Geometry: final body of the model. Coordinates: model frame, mm. A direction names the side the tool comes from. Coordinates: 2 decimals unless noted, no trailing zeros. Loops run counter-clockwise (first coordinate to the right, second up) from the corner with the lowest first, then second, coordinate; pieces in that order, holes last. Notation, with made-up numbers: M -9,12 L -1,12 A24 cw -1,38 Z; hole C 53,-24.5 d1. An arc over 180 degrees is marked long. Write each question's results on one line, items separated by ' | '. Start each with the question number.
from build123d import *

# Parameters (mm, degrees)
F0_W     = 108.312868
F0_H     = 138.248578
F1_DEPTH = 50.8
F2_W     = 90.351426
F2_H     = 123.008572
F3_DEPTH = 110.998
F4_W     = 16.872856
F4_H     = 12.51857
F5_DEPTH = 66.802
F6_DEPTH = 162.56
F7_R     = 9.446924
F8_DEPTH = 123.952
F9_DEPTH = 117.602


with BuildPart() as f1:
    # F0 (on Top) → F1 (new body)
    with BuildSketch(Plane.XY):
        Rectangle(F0_W, F0_H)
    extrude(amount=F1_DEPTH)

    # F2 (on Top) → F3 (cut)
    with BuildSketch(Plane.XY):
        Rectangle(F2_W, F2_H)
    extrude(amount=F3_DEPTH, mode=Mode.SUBTRACT)

    # F4 (on Right) → F5 (cut)
    with BuildSketch(Plane.YZ):
        with Locations((0, 44.631429)):
            Rectangle(F4_W, F4_H)
    extrude(amount=-F5_DEPTH, mode=Mode.SUBTRACT)

    # F4 (on Right) → F6 (cut)
    with BuildSketch(Plane.YZ):
        with Locations((0, 44.631429)):
            Rectangle(F4_W, F4_H)
    extrude(amount=F6_DEPTH, mode=Mode.SUBTRACT)

    # F7 (on Front) → F8 (cut)
    with BuildSketch(Plane.XZ):
        with Locations((0, 27.486429)):
            Circle(F7_R)
    extrude(amount=F8_DEPTH, mode=Mode.SUBTRACT)

    # F7 (on Front) → F9 (cut)
    with BuildSketch(Plane.XZ):
        with Locations((0, 27.486429)):
            Circle(F7_R)
    extrude(amount=-F9_DEPTH, mode=Mode.SUBTRACT)


solid = f1.part
Item 1: Section A-A, the plane x = 42. Return loops of the section in (y, z), plus the area to 3 significant figures.
Item 2: Set-up query: faces 1 (the cylindrical face through (-1.23, -65.261, 36.853)), 2 (the flat face through (45.176, -1, 25)), 3 (the flat face through (-50, 0, 38.372)). Return all of +Z, -Z, +X, -X, +Y, -Y with unobstructed straight access to the full face (end or side cutting, diameter ignored); none if empty.
Item 3: Pull-direction query (Y, two-part tool) for faces 4 (the flat face through (-50, -8.436, 44)), 5 (the flat face through (-54.156, -1, 25)), 6 (the flat face through (-1, -69.124, 14)); classes: released by +Y, released by -Y, zero draft, split by the parting line, or undercut.
Item 4: Section C-C, the plane y = 26. Return loops of the section in (x, z), plus the area to 3 significant figures.
Item 5: Ray query, L1, parallel to Y at x = 38.5, z = 47.5; L2, parallel to Z at x = 0, y = 65; L3, parallel to X at y = 18.5, z = 10. Return the intervals inside material, ascending. Write a range as [from, to].
Item 6: Section D-D, the plane x = 0. Return loops of the section in (y, z).
Item 7: Contact query for flat-ended pins moving along their axis: P1, Ø21.5, axis at x = 0, z = 27.49, coming from the -Y side; P2, Ø7, axis at x = -48, y = -2, coming from the +Z side. Output: stop coordinate, or through.
Item 8: Section B-B, the plane z = 13. Return loops of the section in (x, y).
Solutions:
1) outline: M -69.12,0 L -61.5,0 L -61.5,50.8 L -69.12,50.8 Z; M 61.5,0 L 69.12,0 L 69.12,50.8 L 61.5,50.8 Z | area: 774 mm²
2) face 1: +Y, -Y | face 2: +Z, -Z | face 3: +Z, +X, -X
3) face 4: undercut | face 5: zero draft | face 6: released by -Y
4) outline: M -54.16,0 L -45.18,0 L -45.18,50.8 L -54.16,50.8 Z; M 45.18,0 L 54.16,0 L 54.16,50.8 L 45.18,50.8 Z | area: 912 mm²
5) L1: y = [-69.12, -61.5], [61.5, 69.12] | L2: z = [0, 18.04], [36.93, 50.8] | L3: x = [-54.16, -45.18], [45.18, 54.16]
6) outline: M -69.12,0 L -61.5,0 L -61.5,18.04 L -69.12,18.04 Z; M -69.12,36.93 L -61.5,36.93 L -61.5,50.8 L -69.12,50.8 Z; M 61.5,0 L 69.12,0 L 69.12,18.04 L 61.5,18.04 Z; M 61.5,36.93 L 69.12,36.93 L 69.12,50.8 L 61.5,50.8 Z
7) P1: stops at y = -69.12 | P2: stops at z = 38.37
8) outline: M -54.16,-69.12 L 54.16,-69.12 L 54.16,69.12 L -54.16,69.12 Z; hole M -45.18,-61.5 L 45.18,-61.5 L 45.18,61.5 L -45.18,61.5 Z
